Can you work these out from the model? Positions are in its coordinate system, mm. A direction names the side the tool comes from. Round coordinates to 2 decimals unless told otherwise and drop trailing zeros. One line per item, written item: value. Start each with the question number.
(1) I'm going to push flat-ended pins straight in: pin 1 Ø2 at (y, z) = (9, 6) entering from -X; pin 2 Ø5 at (y, z) = (27, 16.5) entering from +X; pin 3 Ø10 at (x, y) = (6.93, 4) entering from +Z; pin 4 Ø2 at (x, y) = (6.93, 4) entering from -Z. Where does each tip first touch, or does it pass through?
(2) On a 3-axis mill with a long thin cutter (end or side, diameter ignored), from which of +Z, -Z, +X, -X, +Y, -Y can I reach the whole of each face in a straight line? I mean faces 4 (the face through (16, -16, 27)), 5 (the face through (-8, 3, 4)), 6 (the face through (-5.754, -9.784, 11.056)). Say none if no direction works.
(3) If I drill on L1, parallel to Y at x = 1.5, z = 2; L2, parallel to X at y = 3, z = 10.5; L3, parallel to Z at x = 15.5, y = -4.5, over which ranges is the centre line in solid material (lowest first)? Write a range as from..to.
(4) Thinking about a two-plate mould opening in X: for faces 1 (the face through (-4.88, 37.18, 26.75)), 2 (the face through (8, 9, 15)), 3 (the face through (-1, 9, 0)), which applies, +X half, -X half, draft (parallel to the pull), parting line (faces both ways), or undercut?
from build123d import *

# Parameters (mm, degrees)
ESQUISSE1_R              = 37.5
ESQUISSE1_R_2            = 3.25
BOSS_EXTRU_1_DEPTH       = 15
ESQUISSE2_R              = 37.5
ESQUISSE2_R_2            = 18.85
BOSS_EXTRU_2_DEPTH       = 12
ENL_V_MAT_EXTRU_9_DEPTH  = 8
CHANFREIN1_SIZE          = 1
ESQUISSE11_R             = 1.25
ENL_V_MAT_EXTRU_10_DEPTH = 60.510503275
ESQUISSE12_R             = 4.25
ENL_V_MAT_EXTRU_11_DEPTH = 4


with BuildPart() as part:
    # Esquisse1 → Boss.-Extru.1 (new body)
    with BuildSketch(Plane.XY):
        Circle(ESQUISSE1_R)
        Circle(ESQUISSE1_R_2, mode=Mode.SUBTRACT)
    extrude(amount=BOSS_EXTRU_1_DEPTH)

    # Esquisse2 → Boss.-Extru.2 (add)
    with BuildSketch(Plane.XY.offset(15)):
        Circle(ESQUISSE2_R)
        Circle(ESQUISSE2_R_2, mode=Mode.SUBTRACT)
    extrude(amount=BOSS_EXTRU_2_DEPTH)

    # Esquisse9 → Enlèv. mat.-Extru.9 (cut)
    with BuildSketch(Plane.XY.offset(15)):
        Polygon((11.35, -6.552925555), (11.35, 6.552925555), (0, 13.105851111), (-11.35, 6.552925555), (-11.35, -6.552925555), (0, -13.105851111), align=None)
    extrude(amount=-ENL_V_MAT_EXTRU_9_DEPTH, mode=Mode.SUBTRACT)

    # Chanfrein1
    chanfrein1_edges = [part.edges().sort_by_distance(p)[0] for p in [
        (-18.85, 0, 27),
    ]]
    chamfer(chanfrein1_edges, length=CHANFREIN1_SIZE)

    # Esquisse10 → Enlèvement de matière-Révolution1 (revolve, cut)
    with BuildSketch(Plane(origin=(0, 0, 0), x_dir=(0, 0, -1), z_dir=(1, 0, 0)), mode=Mode.PRIVATE) as enl_vement_de_mati_re_r_volution1_sk:
        with BuildLine():
            Line((-26.5, 37.5), (-0.5, 37.5))
            Line((-0.5, 37.5), (-1.5, 35.5))
            ThreePointArc((-1.5, 35.5), (-13.5, 36.5), (-25.5, 35.5))
            Line((-25.5, 35.5), (-26.5, 37.5))
        make_face()
    revolve(enl_vement_de_mati_re_r_volution1_sk.sketch.rotate(Axis((0, 0, 0), (0, 0, 1)), 90), axis=Axis((0, 0, 0), (0, 0, 1)), mode=Mode.SUBTRACT)

    # Esquisse11 → Enlèv. mat.-Extru.10 (cut, through all)
    with BuildSketch(Plane(origin=(0, 0, 0), x_dir=(-1, 0, 0), z_dir=(0, 0, -1))):
        with Locations((-6.92820323, 4)):
            Circle(ESQUISSE11_R)
        with Locations((6.92820323, 4)):
            Circle(ESQUISSE11_R)
        with Locations((0, -8)):
            Circle(ESQUISSE11_R)
    extrude(amount=-ENL_V_MAT_EXTRU_10_DEPTH, mode=Mode.SUBTRACT)

    # Esquisse12 → Enlèv. mat.-Extru.11 (cut)
    with BuildSketch(Plane(origin=(0, 0, 0), x_dir=(-1, 0, 0), z_dir=(0, 0, -1))):
        with Locations((-6.92820323, 4)):
            Circle(ESQUISSE12_R)
        with Locations((6.92820323, 4)):
            Circle(ESQUISSE12_R)
        with Locations((0, -8)):
            Circle(ESQUISSE12_R)
    extrude(amount=-ENL_V_MAT_EXTRU_11_DEPTH, mode=Mode.SUBTRACT)


solid = part.part
Established:
1. pin 1: x = -35.24
1. pin 2: x = 26.98
1. pin 3: z = 15
1. pin 4: through
2. face 4: +Z, +X, -X, +Y, -Y
2. face 5: -Z
2. face 6: +Z
3. L1: -35.55..-11.98, -4.02..-2.88, 2.88..35.55
3. L2: -36.31..-11.35, 11.35..36.31
3. L3: 0..15
4. face 1: parting line
4. face 2: undercut
4. face 3: draft
